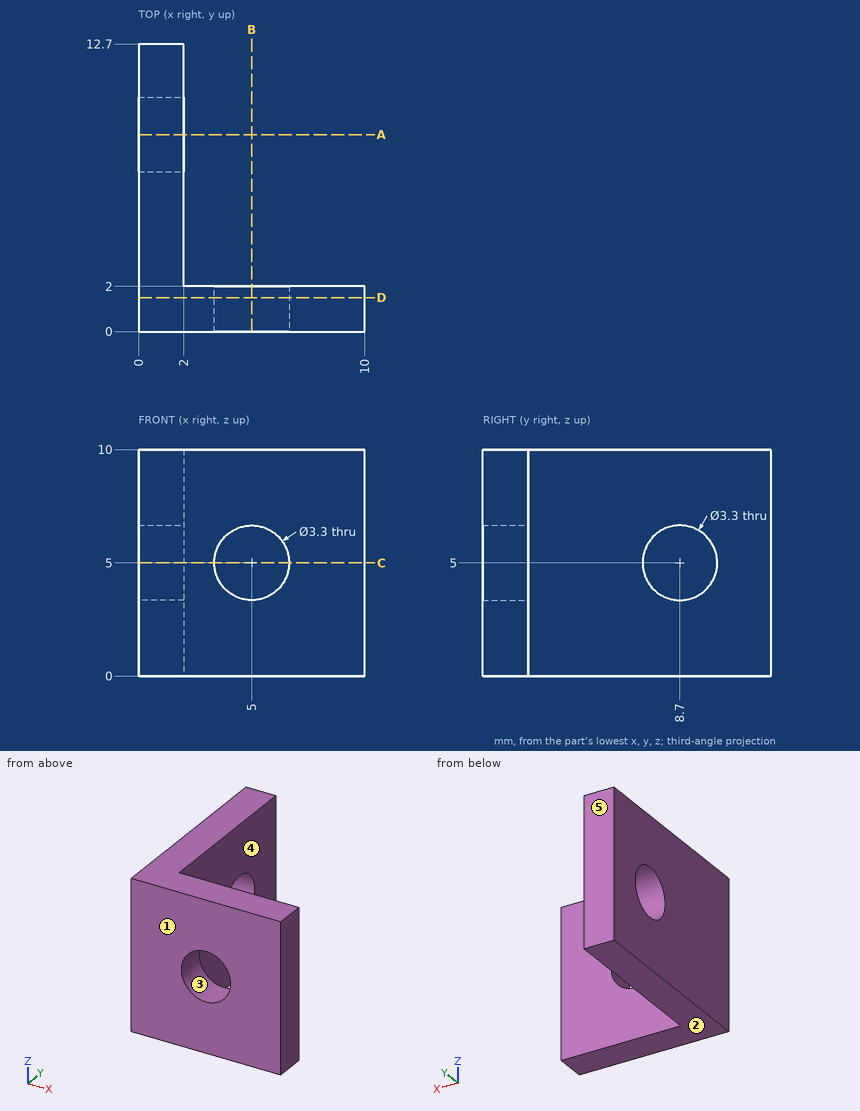
Part print with two shaded views. Sizes in mm from the minimum x, y, z corner. A direction names the side the tool comes from. Round coordinates to 2 decimals unless told otherwise and drop trailing zeros. Loops run counter-clockwise (first coordinate to the right, second up) from the corner with the lowest first, then second, coordinate; pieces in that order, holes last. Notation, with made-up numbers: M -33,-22 L 6,-22 A27 ccw 6,12 Z; hole C 23,-19.5 d8. An arc over 180 degrees is marked long. Return JSON: item names as keys, results as strings. Group by question number.
(1) Drop flat-ended pins along their axis: P1, Ø2, axis at y = 8.7, z = 5, coming from the +X side; P2, Ø4, axis at x = 5.5, z = 5, coming from the +Y side; P3, Ø6, axis at y = 8, z = 6, coming from the -X side; P4, Ø3, axis at y = 5, z = 1.5, coming from the +X side. Give the stop position or say it passes through.
(2) Mould opens along Z. For the marked faces 1, 2 and 3 say: +Z half, -Z half, draft (parallel to the pull), parting line (faces both ways), or undercut.
(3) Wall check: probe 1 along Z at (x, y) = (5, 0.7); probe 2 along Y at (x, z) = (1.25, 5); probe 3 along X at (y, z) = (4.25, 8). Give the ranges that are in metal, low to high. Write a range as [from, to].
(4) Saw through at C-C, the plane z = 5. List the corners of the cut face in (x, y).
(5) Saw through at A-A, the plane y = 8.7. List the corners of the cut face in (x, z), and give its area (3 significant figures).
(6) Tool access for the marked faces 4 and 5: list every direction of +Z, -Z, +X, -X, +Y, -Y with a clear straight run to the whole face (end or side of a thin tool).
(7) Saw through at D-D, the plane y = 1.5. List the corners of the cut face in (x, z).
Answer list:
{
 "1": {"P1": "through", "P2": "y = 2", "P3": "x = 0", "P4": "x = 2"},
 "2": {"face 1": "draft", "face 2": "-Z half", "face 3": "undercut"},
 "3": {"probe 1": "[0, 3.35], [6.65, 10]", "probe 2": "[0, 7.05], [10.35, 12.7]", "probe 3": "[0, 2]"},
 "4": {"outline": "M 0,0 L 3.35,0 L 3.35,2 L 2,2 L 2,7.05 L 0,7.05 Z; M 0,10.35 L 2,10.35 L 2,12.7 L 0,12.7 Z; M 6.65,0 L 10,0 L 10,2 L 6.65,2 Z"},
 "5": {"outline": "M 0,0 L 2,0 L 2,3.35 L 0,3.35 Z; M 0,6.65 L 2,6.65 L 2,10 L 0,10 Z", "area": "13.4 mm2"},
 "6": {"face 4": "+Z, -Z, +X, +Y", "face 5": "+Z, -Z, +X, -X, +Y"},
 "7": {"outline": "M 0,0 L 10,0 L 10,10 L 0,10 Z; hole C 5,5 d3.3"}
}
